The listing builds one solid part. Answer for the finished solid, in the listing's coordinates (mm). A direction names the side the tool comes from. Coordinates: 2 decimals unless noted, no trailing zeros. Write each loop counter-clockwise with the first axis right and the second up, starting at its lowest first coordinate (ties: lowest second). Pieces come first, ordered by that corner, then holes.
(1) For a pull along X with two mould halves and no side action, classify faces 4 (the flat face through (145.062, 13, 1)), 5 (the flat face through (145.062, 81, 1)), 6 (the flat face through (10.762, 27, 1)), 7 (the flat face through (81, 47, 3)) as +X half, -X half, draft (parallel to the pull), parting line (faces both ways), or undercut.
(2) Straight lines are drawn through the part: line 1 (X direction, y = 15, z = 1.2); line 2 (Y direction, x = 50.5, z = 1.85); line 3 (X direction, y = 27.5, z = 2). For each, find the intervals that lie inside material, in ascending order.
(3) Which of the six approach directions +Z, -Z, +X, -X, +Y, -Y give full straight-line access (tool end or side, diameter ignored) to faces 1 (the flat face through (154, 17.217, 1)), 2 (the flat face through (22, 14.217, 1)), 3 (the flat face through (154, 76.217, 1))?
(4) Given P1, Ø0.9, axis at y = 27, z = 1.5, coming from the -X side; P2, Ø0.8, axis at x = 154, z = 1.5, coming from the -Y side; P3, Ø1.5, axis at y = 14.5, z = 1, coming from the +X side, each flat-ended and moving along its own axis, determine where each tip first touches the part or whether it passes through.
(5) The part is cut by section B-B on x = 30.5. Determine the outline of the cut face in (y, z).
from build123d import *

# Parameters (mm, degrees)
SALIENTE_EXTRUIR1_DEPTH = 3
CROQUIS8_W              = 3
CROQUIS8_H              = 64.999858303
CORTAR_EXTRUIR2_DEPTH   = 0.7
CROQUIS10_W             = 2
CROQUIS10_H             = 30
SALIENTE_EXTRUIR3_DEPTH = 3
REDONDEO2_R             = 60


with BuildPart() as part:
    # Croquis1 → Saliente-Extruir1 (new body)
    with BuildSketch(Plane.XY):
        with BuildLine():
            Line((153.062162769, 17.216958542), (155.56216277, 17.216958542))
            Line((155.56216277, 17.216958542), (155.56216277, 76.216816844))
            Line((155.56216277, 76.216816844), (153.062162769, 76.216816844))
            Line((153.062162769, 76.216816844), (153.062162769, 82.216816846))
            ThreePointArc((153.062162769, 82.216816846), (149.062162768, 84.216694386), (145.062162767, 82.216816846))
            Line((145.062162767, 82.216816846), (145.062162767, 79.216816845))
            Line((145.062162767, 79.216816845), (36.062088373, 79.225159863))
            Line((36.062088373, 79.225159863), (36.062088373, 79.770603401))
            ThreePointArc((36.062088373, 79.770603401), (36.039039485, 79.834466742), (35.980517846, 79.868890504))
            Line((35.980517846, 79.868890504), (35.154268939, 80.023817566))
            ThreePointArc((35.154268939, 80.023817566), (35.062123149, 80.032382053), (34.969977306, 80.023818147))
            Line((34.969977306, 80.023818147), (34.143694323, 79.868890087))
            ThreePointArc((34.143694323, 79.868890087), (34.085172266, 79.834466452), (34.062123176, 79.770602869))
            Line((34.062123176, 79.770602869), (34.062123176, 79.216816845))
            Line((34.062123176, 79.216816845), (10.06212317, 79.216816845))
            Line((10.06212317, 79.216816845), (10.06212317, 14.216958542))
            Line((10.06212317, 14.216958542), (34.043728806, 14.216958542))
            Line((34.043728806, 14.216958542), (34.043728806, 13.671515004))
            ThreePointArc((34.043728806, 13.671515004), (34.066777694, 13.607651663), (34.125299333, 13.573227901))
            Line((34.125299333, 13.573227901), (34.95154824, 13.418300839))
            ThreePointArc((34.95154824, 13.418300839), (35.04369403, 13.409736352), (35.135839873, 13.418300258))
            Line((35.135839873, 13.418300258), (35.962122856, 13.573228317))
            ThreePointArc((35.962122856, 13.573228317), (36.020644913, 13.607651952), (36.043694003, 13.671515536))
            Line((36.043694003, 13.671515536), (36.043694003, 14.22530156))
            Line((36.043694003, 14.22530156), (145.062162767, 14.216958542))
            Line((145.062162767, 14.216958542), (145.062162767, 11.216958541))
            ThreePointArc((145.062162767, 11.216958541), (149.062162768, 9.21695854), (153.062162769, 11.216958541))
            Line((153.062162769, 11.216958541), (153.062162769, 17.216958542))
        make_face()
    extrude(amount=SALIENTE_EXTRUIR1_DEPTH)

    # Croquis8 → Cortar-Extruir2 (cut)
    with BuildSketch(Plane.ZY.offset(-10.06212317)):
        with Locations((1.5, 46.716887694)):
            Rectangle(CROQUIS8_W, CROQUIS8_H)
    extrude(amount=-CORTAR_EXTRUIR2_DEPTH, mode=Mode.SUBTRACT)

    # Croquis10 → Saliente-Extruir3 (add)
    with BuildSketch(Plane(origin=(0, 0, 0), x_dir=(-1, 0, 0), z_dir=(0, 0, -1))):
        with Locations((-9.76212317, 54.216816845)):
            Rectangle(CROQUIS10_W, CROQUIS10_H)
    extrude(amount=-SALIENTE_EXTRUIR3_DEPTH)

    # Redondeo2
    # the kernel refuses this fillet: 60 mm, written as the material it takes off along each edge
    with BuildSketch(Plane(origin=(8.76212317, 69.216816845, -38.405728739), x_dir=(1, 0, 0), z_dir=(0, 0, 1))) as redondeo2_piece_1:
        with BuildLine():
            CenterArc((60, -15.362291496), REDONDEO2_R, 165.164888418, 14.835111582)
            Line((0, -15.362291496), (0, 0))
            Line((0, 0), (2, 0))
        make_face()
    extrude(amount=79.811457479, mode=Mode.SUBTRACT)
    with BuildSketch(Plane(origin=(8.76212317, 39.216816845, -38.405728739), x_dir=(0, 1, 0), z_dir=(0, 0, 1))) as redondeo2_piece_2:
        with BuildLine():
            CenterArc((15.362291496, -60), REDONDEO2_R, 90, 14.835111582)
            Line((0, -2), (0, 0))
            Line((0, 0), (15.362291496, 0))
        make_face()
    extrude(amount=79.811457479, mode=Mode.SUBTRACT)


solid = part.part
Model answer:
1. face 4: undercut
1. face 5: undercut
1. face 6: -X half
1. face 7: draft
2. line 1: x = 10.76 to 153.06
2. line 2: y = 14.22 to 79.22
2. line 3: x = 10.76 to 155.56
3. face 1: +Z, -Z, +X, -Y
3. face 2: +Z, -Z, -X, -Y
3. face 3: +Z, -Z, +X, +Y
4. P1: stops at x = 10.76
4. P2: stops at y = 17.22
4. P3: stops at x = 153.06
5. outline: (14.22, 0) - (79.22, 0) - (79.22, 3) - (14.22, 3) - close
